Geometry: final body of the model. Coordinates: model frame, mm. Coordinates: 2 decimals unless noted, no trailing zeros. Loops run counter-clockwise (first coordinate to the right, second up) from the corner with the lowest first, then second, coordinate; pieces in that order, holes last. Notation, with made-up numbers: (-18, -38.5) - (5, -38.5) arc R22 ccw to (5, -19.5) - close; hole circle Ø4 at (56, 87.25). An arc over 180 degrees is marked (long way). Answer in a Markdown table with one row per item.
from build123d import *

# Parameters (mm, degrees)
SKETCH1_W                = 40
SKETCH1_H                = 40
BOSS_EXTRUDE1_DEPTH      = 20
SURFACE_EXTRUDE1_1_BACK  = 50
SURFACE_EXTRUDE1_1_DEPTH = 100


with BuildPart() as part:
    # Sketch1 → Boss-Extrude1 (new body)
    with BuildSketch(Plane.XY):
        with Locations((20, 20)):
            Rectangle(SKETCH1_W, SKETCH1_H)
    extrude(amount=BOSS_EXTRUDE1_DEPTH)

    # SurfaceCut1: cut with a surface, the side it looks to stays
    # Surface-Extrude1: a surface, the sketch's curves swept straight by 100 mm
    with BuildLine(Plane(origin=(0, 0, 0), x_dir=(0, 0, -1), z_dir=(1, 0, 0)).offset(-SURFACE_EXTRUDE1_1_BACK), mode=Mode.PRIVATE) as surface_extrude1_1_path:
        Line((-5, -10), (-15, 50))
    surface_extrude1_1 = Shell.extrude(surface_extrude1_1_path.wire(), (1 * SURFACE_EXTRUDE1_1_DEPTH, 0 * SURFACE_EXTRUDE1_1_DEPTH, 0 * SURFACE_EXTRUDE1_1_DEPTH))
    split(bisect_by=surface_extrude1_1, keep=Keep.TOP)


solid = part.part
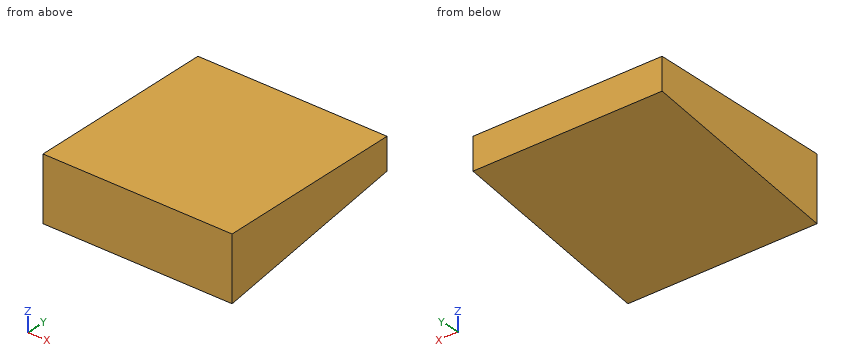
(1) Cut plane A-A on y = 36.5. Output: boundary loops of the cut face in (x, z), then the cut area to 3 significant figures.
Verdict:
| item | result |
|---|---|
| outline | (0, 12.75) - (40, 12.75) - (40, 20) - (0, 20) - close |
| area | 290 mm² |
(2) Ray query, probe 1 along Z at (x, y) = (2, 25); probe 2 along Z at (x, y) = (19, 14.5). Return the intervals inside material, ascending.
Verdict:
| item | result |
|---|---|
| probe 1 | z = 10.83 to 20 |
| probe 2 | z = 9.08 to 20 |
(3) Cut plane B-B on z = 9.5. Output: boundary loops of the cut face in (x, y).
Verdict:
| item | result |
|---|---|
| outline | (0, 0) - (40, 0) - (40, 17) - (0, 17) - close |
(4) First-contact query: pin 1 Ø12 at (x, y) = (5, 12.5) entering from -Z. Flat tip, straight axial feed; report the tip coordinate or a pass-through.
Verdict:
| item | result |
|---|---|
| pin 1 | stops at z = 7.75 |
